Model file for the job. Use its own axes, mm. Face numbers are marked on the shaded views. A direction names the side the tool comes from. Coordinates: 2 decimals unless noted, no trailing zeros. Write each loop counter-clockwise with the first axis right and the second up, starting at its lowest first coordinate (ties: lowest second). Pieces come first, ordered by that corner, then holes. Notation, with made-up numbers: M 31.5,-31.5 L 64.5,-31.5 A21 cw 64.5,-8.5 Z; hole C 26.5,33 d9. An arc over 180 degrees is marked long. Use CSV: the item, a comma, the result in double quotes. Start each with the question number.
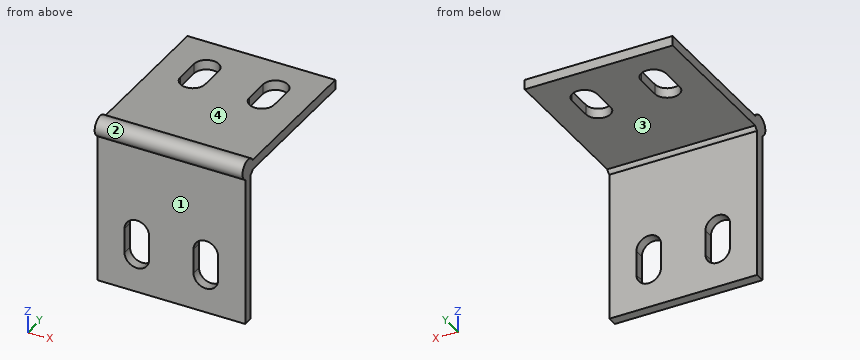
Autodesk Inventor part; units mm, degrees
ref_plane "YZ Plane" through (0, 0, 0) normal (1, 0, 0) x (0, 1, 0)
ref_plane "XZ Plane" through (0, 0, 0) normal (0, 1, 0) x (-1, 0, 0)
ref_plane "XY Plane" through (0, 0, 0) normal (0, 0, 1) x (1, 0, 0)
sketch "Sketch1" plane through (0, 0, 0) normal (1, 0, 0) x (0, 1, 0)
  line L0 (1.7321, 1) -> (32, 1)
  line L1 (32, 1) -> (32, -1)
  line L2 (32, -1) -> (1.7321, -1)
  line L3 (1.7321, 1) -> (32, 1)
  line L4 (32, 1) -> (32, -1)
  line L5 (32, -1) -> (1.7321, -1)
  line L6 (1, -1.7273) -> (1, -31.9952)
  line L7 (1, -31.9952) -> (-1, -31.9952)
  line L8 (-1, -31.9952) -> (-1, -1.7273)
  arc A0 (1, -1.7321) -> (1.7321, -1) centre (0, 0) ccw
  arc A1 (1.7321, 1) -> (-1, -1.7321) centre (0, 0) ccw
  dimension "d6" = 2
  dimension "d8" = 30.2679
  dimension "d9" = 30.2679
  dimension "d33" = 2
extrude "Extrusion1" add sketch "Sketch1" along normal blind 30
sketch "Sketch2" plane through (0, 1, -1.7321) normal (0, 1, 0) x (1, 0, 0)
  line L0 (8, 22.7632) -> (8, 17.7632) construction
  line L1 (10.5, 22.7632) -> (10.5, 17.7632)
  line L2 (5.5, 17.7632) -> (5.5, 22.7632)
  arc A0 (10.5, 22.7632) -> (5.5, 22.7632) centre (8, 22.7632) ccw
  arc A1 (5.5, 17.7632) -> (10.5, 17.7632) centre (8, 17.7632) ccw
  line L3 (22, 22.7632) -> (22, 17.7632) construction
  line L4 (24.5, 22.7632) -> (24.5, 17.7632)
  line L5 (19.5, 17.7632) -> (19.5, 22.7632)
  arc A2 (24.5, 22.7632) -> (19.5, 22.7632) centre (22, 22.7632) ccw
  arc A3 (19.5, 17.7632) -> (24.5, 17.7632) centre (22, 17.7632) ccw
  line L6 (0, 30.2632) -> (30, 30.2632)
  line L7 (30, 30.2632) -> (30, 0)
  line L8 (0, 30.2632) -> (0, 0)
  point P0 (0, -1.7321)
  point P1 (8, 20.2632)
  point P2 (22, 20.2632)
  dimension "d12" = 5
  dimension "d13" = 10
  dimension "d14" = 5
  dimension "d15" = 10
  dimension "d16" = 10
  dimension "d17" = 10
  dimension "d18" = 8
  dimension "d19" = 8
extrude "Extrusion2" cut sketch "Sketch2" against normal blind 10
sketch "Sketch3" plane through (0, 1.7321, -1) normal (0, 0, -1) x (-1, 0, 0)
  line L0 (-5.5, -0.7321) -> (-10.5, -0.7321)
  line L1 (-10.5, -0.7321) -> (-5.5, -0.7321)
  line L2 (-19.5, -0.7321) -> (-24.5, -0.7321)
  line L3 (-24.5, -0.7321) -> (-19.5, -0.7321)
  line L4 (0, -0.7321) -> (-30, -0.7321)
  line L5 (0, -0.7321) -> (-30, -0.7321)
  line L6 (0, 0) -> (0, 30.2679)
  line L7 (0, 30.2679) -> (-30, 30.2679)
  line L8 (-30, 0) -> (-30, 30.2679)
  line L9 (0, 0) -> (-30, 0)
  line L10 (-5.5, -0.7321) -> (-10.5, -0.7321)
  line L11 (-10.5, -0.7321) -> (-5.5, -0.7321)
  line L12 (-19.5, -0.7321) -> (-24.5, -0.7321)
  line L13 (-24.5, -0.7321) -> (-19.5, -0.7321)
  line L14 (0, -0.7321) -> (-30, -0.7321)
  line L15 (0, -0.7321) -> (-30, -0.7321)
  line L16 (-5.5, -0.7321) -> (-10.5, -0.7321)
  line L17 (-10.5, -0.7321) -> (-5.5, -0.7321)
  line L18 (-19.5, -0.7321) -> (-24.5, -0.7321)
  line L19 (-24.5, -0.7321) -> (-19.5, -0.7321)
  line L20 (0, -0.7321) -> (-30, -0.7321)
  line L21 (0, -0.7321) -> (-30, -0.7321)
  line L22 (-5.5, -0.7321) -> (-10.5, -0.7321)
  line L23 (-10.5, -0.7321) -> (-5.5, -0.7321)
  line L24 (-19.5, -0.7321) -> (-24.5, -0.7321)
  line L25 (-24.5, -0.7321) -> (-19.5, -0.7321)
  line L26 (0, -0.7321) -> (-30, -0.7321)
  line L27 (0, -0.7321) -> (-30, -0.7321)
  line L28 (-22, 17.7679) -> (-22, 22.7679) construction
  line L29 (-24.5, 17.7679) -> (-24.5, 22.7679)
  line L30 (-19.5, 22.7679) -> (-19.5, 17.7679)
  arc A0 (-24.5, 17.7679) -> (-19.5, 17.7679) centre (-22, 17.7679) ccw
  arc A1 (-19.5, 22.7679) -> (-24.5, 22.7679) centre (-22, 22.7679) ccw
  line L31 (-8, 17.7679) -> (-8, 22.7679) construction
  line L32 (-10.5, 17.7679) -> (-10.5, 22.7679)
  line L33 (-5.5, 22.7679) -> (-5.5, 17.7679)
  arc A2 (-10.5, 17.7679) -> (-5.5, 17.7679) centre (-8, 17.7679) ccw
  arc A3 (-5.5, 22.7679) -> (-10.5, 22.7679) centre (-8, 22.7679) ccw
  point P0 (0, -1.7321)
  point P1 (-22, 20.2679)
  point P2 (-8, 20.2679)
  dimension "d23" = 10
  dimension "d24" = 5
  dimension "d25" = 10
  dimension "d26" = 8
  dimension "d27" = 10
  dimension "d28" = 5
  dimension "d29" = 8
  dimension "d30" = 10
extrude "Extrusion3" cut sketch "Sketch3" against normal blind 10 contours L29 A1 L30 A0 | L32 A3 L33 A2
properties part number "Hinge"
1) Band-saw the part on B-B on x = 8. List the corners of the cut face in (y, z).
2) Wall check: L1, parallel to X at y = 18, z = 0.5; L2, parallel to Z at x = 19.75, y = 7.5. Give the ranges that are in metal, low to high. Write a range as [from, to].
3) Band-saw the part on A-A on y = 18. List the corners of the cut face in (x, z).
4) Band-saw the part on C-C on y = 0. List the corners of the cut face in (x, z), then the cut area to 3 significant figures.
5) Drop flat-ended pins along their axis: P1, Ø5, axis at x = 6.5, y = 7, coming from the +Z side; P2, Ø5, axis at x = 25, y = 13, coming from the -Z side; P3, Ø6, axis at x = 24, z = -10.5, coming from the +Y side. Give the stop position or say it passes through.
6) Band-saw the part on D-D on x = 3. List the corners of the cut face in (y, z).
7) Tool access for the marked faces 1, 2, 3 and 4: list every direction of +Z, -Z, +X, -X, +Y, -Y with a clear straight run to the whole face (end or side of a thin tool).
Findings below:
1,outline,"M -1,-32 L 1,-32 L 1,-27 L -1,-27 Z; M -1,-17 L 1,-17 L 1,-1.73 A2 ccw 1.73,-1 L 17,-1 L 17,1 L 1.73,1 A2 ccw long -1,-1.73 Z; M 27,-1 L 32,-1 L 32,1 L 27,1 Z"
2,L1,"x = [0, 6], [10, 20], [24, 30]"
2,L2,"z = [-1, 1]"
3,outline,"M 0,-1 L 6,-1 L 6,1 L 0,1 Z; M 10,-1 L 20,-1 L 20,1 L 10,1 Z; M 24,-1 L 30,-1 L 30,1 L 24,1 Z"
4,outline,"M 0,-32 L 30,-32 L 30,2 L 0,2 Z; hole M 5.5,-24.5 A2.5 ccw 10.5,-24.5 L 10.5,-19.5 A2.5 ccw 5.5,-19.5 Z; hole M 19.5,-24.5 A2.5 ccw 24.5,-24.5 L 24.5,-19.5 A2.5 ccw 19.5,-19.5 Z"
4,area,"931 mm2"
5,P1,"stops at z = 1"
5,P2,"stops at z = -1"
5,P3,"stops at y = 1"
6,outline,"M -1,-32 L 1,-32 L 1,-1.73 A2 ccw 1.73,-1 L 32,-1 L 32,1 L 1.73,1 A2 ccw long -1,-1.73 Z"
7,face 1,"-Z, +X, -X, -Y"
7,face 2,"+X, -X"
7,face 3,"-Z, +X, -X, +Y"
7,face 4,"+Z, +X, -X, +Y"
